Design review of the part built by this model. Coordinates are the model's own, in mm. Face numbers are marked on the shaded views. A direction names the side the tool comes from. Coordinates: 2 decimals unless noted, no trailing zeros. Write each loop counter-clockwise with the first axis right and the second up, starting at its lowest first coordinate (ties: lowest second). Pieces come first, ordered by that corner, then holes.
Q1. Mouldability with a two-part tool opening along Y and no side actions: class the marked faces 1, 2 and 3 as pulls with the +Y half, pulls with the -Y half, needs draft (parallel to the pull), parting line crosses it, or undercut.
Q2. Take a section at B-B (y = -115). Give the boundary of the cut face in (x, z).
Q3. Take a section at A-A (z = 0). State how many separate pieces and enclosed holes the cut face has, and give its area (3 significant figures).
Q4. Take a section at C-C (y = -40). Give the boundary of the cut face in (x, z).
Q5. Machinability: for the marked faces 4, 5 and 6, which of the approach directions +Z, -Z, +X, -X, +Y, -Y give a long, thin tool a straight path to every point of the face, cutting with its end or side? Answer none if there is none.
Q6. For probe 1 along Y at (x, z) = (-24.5, -32.5); probe 2 along Z at (x, y) = (0, -115), list the stretches that pass through material, from the lowest coordinate up.
Q7. Insertion check: pin 1 (3 mm diameter, centred on y = -55.5, z = -52.5, fed in from -X); pin 2 (12 mm diameter, centred on x = 40.5, y = -83, fed in from +Z); pin 3 (10 mm diameter, centred on x = -2.5, z = -53, fed in from +Y). Each pin has a flat end and moves straight along its axis. Give the tip position at first contact, or say it passes through.
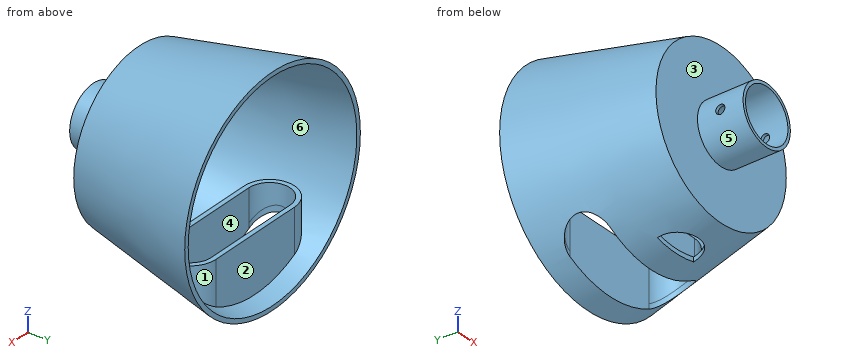
```python
from build123d import *

# Parameters (mm, degrees)
SKETCH1_R               = 75
BOSS_EXTRUDE1_DEPTH     = 100
BOSS_EXTRUDE1_TAPER     = 12
SKETCH3_R               = 70
CUT_EXTRUDE1_DEPTH      = 80
CUT_EXTRUDE1_TAPER      = 12
FILLET1_R               = 10
CUT_EXTRUDE2_DEPTH      = 90
SKETCH5_R               = 19.5
SKETCH5_R_2             = 17.5
BOSS_EXTRUDE2_DEPTH     = 30
SKETCH6_R               = 17.5
CUT_EXTRUDE3_DEPTH      = 30
BOSS_EXTRUDE7_REACH     = 44.651
SKETCH17_R              = 73.5
CUT_EXTRUDE4_DEPTH      = 25
SKETCH18_R              = 3
CUT_EXTRUDE5_DEPTH      = 73.432504542
CUT_EXTRUDE5_DEPTH_BACK = 73.432504542


with BuildPart() as part:
    # Sketch1 → Boss-Extrude1 (new body)
    with BuildSketch(Plane(origin=(0, 0, 0), x_dir=(1, 0, 0), z_dir=(0, 1, 0))):
        Circle(SKETCH1_R)
    extrude(amount=-BOSS_EXTRUDE1_DEPTH, taper=BOSS_EXTRUDE1_TAPER)

    # Sketch3 → Cut-Extrude1 (cut)
    with BuildSketch(Plane(origin=(0, -10, 0), x_dir=(1, 0, 0), z_dir=(0, 1, 0))):
        Circle(SKETCH3_R)
    extrude(amount=-CUT_EXTRUDE1_DEPTH, taper=CUT_EXTRUDE1_TAPER, mode=Mode.SUBTRACT)

    # Fillet1
    fillet1_edges = [part.edges().sort_by_distance(p)[0] for p in [
        (-75, 0, 0),
    ]]
    fillet(fillet1_edges, radius=FILLET1_R)

    # Sketch4 → Cut-Extrude2 (cut)
    with BuildSketch(Plane.XY):
        with BuildLine():
            Line((-15, -70), (15, -70))
            ThreePointArc((15, -70), (0, -85), (-15, -70))
        make_face()
        with BuildLine():
            Line((-32.5, -26.5), (32.5, -26.5))
            ThreePointArc((32.5, -26.5), (46, -40), (32.5, -53.5))
            Line((32.5, -53.5), (-32.5, -53.5))
            ThreePointArc((-32.5, -53.5), (-46, -40), (-32.5, -26.5))
        make_face()
    extrude(amount=-CUT_EXTRUDE2_DEPTH, mode=Mode.SUBTRACT)

    # Sketch5 → Boss-Extrude2 (add)
    with BuildSketch(Plane.XZ.offset(100)):
        Circle(SKETCH5_R)
        Circle(SKETCH5_R_2, mode=Mode.SUBTRACT)
    extrude(amount=BOSS_EXTRUDE2_DEPTH)

    # Sketch6 → Cut-Extrude3 (cut)
    with BuildSketch(Plane.XZ.offset(100)):
        Circle(SKETCH6_R)
    extrude(amount=-CUT_EXTRUDE3_DEPTH, mode=Mode.SUBTRACT)

    # Sketch16 → Boss-Extrude7 (add, up to next)
    with BuildSketch(Plane.XY.offset(-30), mode=Mode.PRIVATE) as boss_extrude7_sk1:
        with BuildLine():
            Line((32.5, -56.5), (-32.5, -56.5))
            ThreePointArc((-32.5, -56.5), (-49, -40), (-32.5, -23.5))
            Line((-32.5, -23.5), (32.5, -23.5))
            ThreePointArc((32.5, -23.5), (49, -40), (32.5, -56.5))
        make_face()
        with BuildLine():
            Line((32.5, -53.5), (-32.5, -53.5))
            ThreePointArc((-32.5, -53.5), (-46, -40), (-32.5, -26.5))
            Line((-32.5, -26.5), (32.5, -26.5))
            ThreePointArc((32.5, -26.5), (46, -40), (32.5, -53.5))
        make_face(mode=Mode.SUBTRACT)
    boss_extrude7_tool1 = extrude(boss_extrude7_sk1.sketch, amount=-BOSS_EXTRUDE7_REACH, mode=Mode.PRIVATE) - part.part
    add(boss_extrude7_tool1.solids().sort_by_distance((0, -55.46593, -30))[0])

    # Sketch17 → Cut-Extrude4 (cut)
    with BuildSketch(Plane(origin=(0, -12.079116908, 0), x_dir=(1, 0, 0), z_dir=(0, 1, 0))):
        Circle(SKETCH17_R)
    extrude(amount=CUT_EXTRUDE4_DEPTH, mode=Mode.SUBTRACT)

    # Sketch18 → Cut-Extrude5 (cut, two sides)
    with BuildSketch(Plane(origin=(0, 0, 0), x_dir=(0, 0, -1), z_dir=(1, 0, 0))) as cut_extrude5_sk:
        with Locations((0, -115)):
            Circle(SKETCH18_R)
    extrude(amount=CUT_EXTRUDE5_DEPTH, mode=Mode.SUBTRACT)
    extrude(cut_extrude5_sk.sketch, amount=-CUT_EXTRUDE5_DEPTH_BACK, mode=Mode.SUBTRACT)


solid = part.part
```
Response:
1. face 1: undercut
1. face 2: pulls with the +Y half
1. face 3: pulls with the -Y half
2. outline: (-19.27, -3) arc R19.5 ccw to (19.27, -3) - (17.24, -3) arc R17.5 cw to (-17.24, -3) - close; (-19.27, 3) - (-17.24, 3) arc R17.5 cw to (17.24, 3) - (19.27, 3) arc R19.5 ccw to start
3. separate pieces: 4
3. enclosed holes: 0
3. area: 1,290 mm2
4. outline: (-49, -40.58) arc R63.62 cw (long way) to (49, -40.58) - (49, -30) - (46, -30) - (46, -48.02) arc R66.5 ccw (long way) to (-46, -48.02) - (-46, -30) - (-49, -30) - close
5. face 4: -Z
5. face 5: -Y
5. face 6: none
6. probe 1: y = -100 to -90, -56.5 to -53.5, -26.5 to -23.5
6. probe 2: z = -19.5 to -17.5, 17.5 to 19.5
7. pin 1: stops at x = -37.4
7. pin 2: stops at z = 46.1
7. pin 3: stops at y = -23.5
